```python
from build123d import *

# Parameters (mm, degrees)
F1_DEPTH = 14
F3_DEPTH = 11
F4_R     = 2.1
F5_DEPTH = 14.001
F6_SIZE2 = 6.5
F6_SIZE  = 8.255
F7_DEPTH = 25.4
F2_W     = 7
F2_H     = 3.5
F8_DEPTH = 10.0010001
F2_R     = 2
F9_DEPTH = 25


# Not quite as in the source:
# - a feature names something its author has since deleted; it is built from what else it names


with BuildPart() as f1:
    # F0 (on Front) → F1 (new body)
    with BuildSketch(Plane.XZ):
        Polygon((10, 21.0440813839), (0, 21.0440813839), (0, 0), (0, -4.3559186161), (10, -4.3559186161), (10, 0), align=None)
    extrude(amount=F1_DEPTH)

    # F2 (on face) → F3 (join)
    with BuildSketch(Plane.YZ.offset(10)):
        with BuildLine():
            Line((0, -3.4542235791), (0, 20.1423863469))
            ThreePointArc((0, 20.1423863469), (-8, 8.3440813839), (0, -3.4542235791))
        make_face()
    extrude(amount=-F3_DEPTH)

    # F4 (on face) → F5 (cut, through all)
    with BuildSketch(Plane.XZ.offset(14)):
        with Locations((5, 8.3440813839)):
            Circle(F4_R)
    extrude(amount=-F5_DEPTH, mode=Mode.SUBTRACT)

    # F6
    f6_edges = [f1.edges().sort_by_distance(p)[0] for p in [
        (5, -14, 21.044081),
    ]]
    f6_side = f1.faces().sort_by_distance((5, -7, 21.044081))[0]
    chamfer(f6_edges, length=F6_SIZE, length2=F6_SIZE2, reference=f6_side)

    # F2 (on face) → F7 (cut)
    with BuildSketch(Plane.YZ.offset(10)):
        with BuildLine():
            Line((0, -3.4542235791), (0, 20.1423863469))
            ThreePointArc((0, 20.1423863469), (-8, 8.3440813839), (0, -3.4542235791))
        make_face()
    extrude(amount=-F7_DEPTH, mode=Mode.SUBTRACT)

    # F2 (on face) → F8 (cut, through all)
    with BuildSketch(Plane.YZ.offset(10)):
        with Locations((-10.5, -2.6059186161)):
            Rectangle(F2_W, F2_H)
    extrude(amount=-F8_DEPTH, mode=Mode.SUBTRACT)

    # F2 (on face) → F9 (cut)
    with BuildSketch(Plane.YZ.offset(10)):
        with BuildLine():
            Line((4.7, 21.0440813839), (1.525, 21.0440813839))
            Line((1.525, 21.0440813839), (1.525, 20.6408035082))
            ThreePointArc((1.525, 20.6408035082), (3.0997454855, 20.9428585265), (4.7, 21.0440813839))
        make_face()
        with BuildLine():
            Line((7.875, 21.0440813839), (4.7, 21.0440813839))
            ThreePointArc((4.7, 21.0440813839), (3.0997454855, 20.9428585265), (1.525, 20.6408035082))
            Line((1.525, 20.6408035082), (1.525, -3.9526407403))
            ThreePointArc((1.525, -3.9526407403), (3.0997454855, -4.2546957586), (4.7, -4.3559186161))
            Line((4.7, -4.3559186161), (7.875, -4.3559186161))
            Line((7.875, -4.3559186161), (7.875, 21.0440813839))
        make_face()
        with BuildLine():
            Line((1.525, -3.9526407403), (1.525, 20.6408035082))
            ThreePointArc((1.525, 20.6408035082), (0.7546215433, 20.4157005311), (0, 20.1423863469))
            Line((0, 20.1423863469), (0, -3.4542235791))
            ThreePointArc((0, -3.4542235791), (0.7546215433, -3.7275377632), (1.525, -3.9526407403))
        make_face()
        with BuildLine():
            ThreePointArc((4.7, -4.3559186161), (3.0997454855, -4.2546957586), (1.525, -3.9526407403))
            Line((1.525, -3.9526407403), (1.525, -4.3559186161))
            Line((1.525, -4.3559186161), (2.607938957, -4.3559186161))
            Line((2.607938957, -4.3559186161), (4.7, -4.3559186161))
        make_face()
        with BuildLine():
            Line((0, -3.4542235791), (0, 20.1423863469))
            ThreePointArc((0, 20.1423863469), (-8, 8.3440813839), (0, -3.4542235791))
        make_face()
        with Locations((-11.0123908797, 3.1440813839)):
            Circle(F2_R)
    extrude(amount=-F9_DEPTH, mode=Mode.SUBTRACT)


solid = f1.part
```
Could you check a few things on this model? Use its own coordinates, in mm. A direction names the side the tool comes from. Round coordinates to 2 decimals unless told otherwise and drop trailing zeros. Loops run counter-clockwise (first coordinate to the right, second up) from the corner with the lowest first, then second, coordinate; pieces in that order, holes last. Notation, with made-up numbers: (-23.5, 55) -> (-15.5, 55) arc R31 ccw to (-15.5, 86) -> close; hole circle Ø9 at (5, 59). An arc over 180 degrees is marked (long way). Put each result on its own line as item: value.
Q1. Which directions (+Z, -Z, +X, -X, +Y, -Y) give clear straight access to the entire face, cutting with the end or side of a thin tool? Please do faces 4 (the flat face through (5, -3, 21.044)), 5 (the flat face through (5, -11, -0.856)).
Checks:
face 4: +Z, +X, -X, +Y, -Y
face 5: -Z, +X, -X, -Y
Q2. I want a section at C-C on z = 1.75. Write out the boundary of the cut face in (x, y).
Checks:
outline: (0, -14) -> (10, -14) -> (10, -12.45) -> (0, -12.45) -> close; (0, -9.58) -> (10, -9.58) -> (10, -6.15) -> (0, -6.15) -> close
Q3. I want a section at B-B on y = -10.5. Write out the boundary of the cut face in (x, z).
Checks:
outline: (0, -0.86) -> (10, -0.86) -> (10, 1.21) -> (0, 1.21) -> close; (0, 5.08) -> (10, 5.08) -> (10, 17.3) -> (0, 17.3) -> close; hole circle Ø4.2 at (5, 8.34)
Q4. I want a section at D-D on x = 2. Write out the boundary of the cut face in (y, z) (3 decimals), and give its area (3 significant figures).
Checks:
outline: (-14, -0.856) -> (-7, -0.856) -> (-7, -4.356) -> (0, -4.356) -> (0, -3.454) arc R12.7 cw to (0, 20.142) -> (0, 21.044) -> (-5.745, 21.044) -> (-14, 14.544) -> close; hole circle Ø4 at (-11.012, 3.144)
area: 155 mm2
Q5. Thinking about a two-plate mould opening in Z: for faces 1 (the cylindrical face through (5.07, -13.01, 3.23)), 2 (the flat face through (5, -7, -3)), 3 (the flat face through (5, -3, -4.356)), which applies, pulls with the +Z half, pulls with the -Z half, needs draft (parallel to the pull), parting line crosses it, or undercut?
Checks:
face 1: undercut
face 2: needs draft
face 3: pulls with the -Z half
Q6. I want a section at A-A on x = 3.75. Write out the boundary of the cut face in (y, z) (3 decimals), and give its area (3 significant figures).
Checks:
outline: (-14, -0.856) -> (-7, -0.856) -> (-7, -4.356) -> (0, -4.356) -> (0, -3.454) arc R12.7 cw to (-7.887, 6.657) -> (-14, 6.657) -> close; (-14, 10.032) -> (-7.887, 10.032) arc R12.7 cw to (0, 20.142) -> (0, 21.044) -> (-5.745, 21.044) -> (-14, 14.544) -> close; hole circle Ø4 at (-11.012, 3.144)
area: 135 mm2
Q7. For pin 1 Ø5 at (x, z) = (5, 8.34) entering from +Y; pin 2 Ø1 at (x, z) = (5.5, -2.5) entering from -Y; pin 3 Ø3 at (y, z) = (-8, 5.5) entering from -X; pin 4 Ø2 at (x, y) = (3, -9) entering from -Z, each with a flat end and sliding along its axis, tell me the tip position at first contact or that it passes through.
Checks:
pin 1: y = -7.75
pin 2: y = -7
pin 3: x = 0
pin 4: z = -0.86
Q8. Please list where these lines run through material, in increasing order: line 1 (Z direction, x = 5, y = -10); line 2 (Z direction, x = 5.5, y = -12.5); line 3 (Y direction, x = 9.5, z = 4.25). Write a range as from..to.
Checks:
line 1: -0.86..1.42, 4.87..6.24, 10.44..17.69
line 2: -0.86..1.81, 4.48..6.3, 10.38..15.73
line 3: -14..-12.68, -9.35..-7.32
